```python
from build123d import *

# Parameters (mm, degrees)
SKETCH1_W             = 10
SKETCH1_H             = 15
BOSS_EXTRUDE1_DEPTH   = 15
M5X0_8_TAPPED_HOLE1_D = 4.2
M5X0_8_TAPPED_HOLE2_D = 4.2


with BuildPart() as part:
    # Sketch1 → Boss-Extrude1 (new body)
    with BuildSketch(Plane.XY):
        Rectangle(SKETCH1_W, SKETCH1_H)
    extrude(amount=BOSS_EXTRUDE1_DEPTH)

    # M5x0.8 Tapped Hole1 (through all)
    with Locations(Plane(origin=(0, 7.5, 0), x_dir=(1, 0, 0), z_dir=(0, 1, 0))):
        with Locations((0, -4)):
            Hole(M5X0_8_TAPPED_HOLE1_D / 2)

    # M5x0.8 Tapped Hole2 (through all)
    with Locations(Plane.ZY.offset(5)):
        with Locations((11, -2.5)):
            Hole(M5X0_8_TAPPED_HOLE2_D / 2)


solid = part.part
```
Here's how the part is built. I have some questions about the finished solid (model axes, mm). Give positions to 0.01 mm unless a question says otherwise; leave off trailing zeros. Order: outer loops, then holes, each group sorted by start corner. A loop starts at its lowest first (then second) coordinate and runs counter-clockwise, first axis right, second up. Notation, with made-up numbers: (31, -5.75) -> (90, -5.75) arc R14 ccw to (90, 16.25) -> close; hole circle Ø9 at (26, 8.5). An arc over 180 degrees is marked (long way). Use CSV: the item, a comma, the result in double quotes. Start each with the question number.
Item 1: Suppose I cut it at D-D (x = -2.5). List the corners of the cut face in (y, z) for me.
Item 2: Suppose I cut it at A-A (y = -2.5). List the corners of the cut face in (x, z) for me, and give its area (3 significant figures).
Item 3: If I drill on probe 1 along Y at (x, z) = (-0.5, 11); probe 2 along Z at (x, y) = (0, 0); probe 3 along Z at (x, y) = (0.5, -1), over which ranges is the centre line in solid material (lowest first)? Write a range as [from, to].
Item 4: Thinking about a two-plate mould opening in Z: for faces 1 (the flat face through (0, 0, 0)), 2 (the cylindrical face through (0.07, -2.41, 13.1)), 3 (the flat face through (0, 7.5, 7)), which applies, pulls with the +Z half, pulls with the -Z half, needs draft (parallel to the pull), parting line crosses it, or undercut?
Item 5: Suppose I cut it at B-B (z = 4). List the corners of the cut face in (x, y) for me, and give its area (3 significant figures).
Item 6: I'm going to push a flat-ended pin straight in: P1, Ø2, axis at x = -0.5, z = 4, coming from the +Y side. Where does the tip first touch, or does it pass through?
Item 7: Suppose I cut it at C-C (x = 0). List the corners of the cut face in (y, z) for me, and give its area (3 significant figures).
Answer block:
1,outline,"(-7.5, 0) -> (7.5, 0) -> (7.5, 15) -> (-7.5, 15) -> close; hole circle Ø4.2 at (-2.5, 11)"
2,outline,"(-5, 0) -> (5, 0) -> (5, 8.9) -> (-5, 8.9) -> close; (-5, 13.1) -> (5, 13.1) -> (5, 15) -> (-5, 15) -> close; hole circle Ø4.2 at (0, 4)"
2,area,"94.1 mm^2"
3,probe 1,"y = [-7.5, -4.6], [-0.4, 7.5]"
3,probe 2,"z = [0, 1.9], [6.1, 15]"
3,probe 3,"z = [0, 1.96], [6.04, 9.53], [12.47, 15]"
4,face 1,"pulls with the -Z half"
4,face 2,"undercut"
4,face 3,"needs draft"
5,outline,"(-5, -7.5) -> (-2.1, -7.5) -> (-2.1, 7.5) -> (-5, 7.5) -> close; (2.1, -7.5) -> (5, -7.5) -> (5, 7.5) -> (2.1, 7.5) -> close"
5,area,"87.0 mm^2"
6,P1,"passes through"
7,outline,"(-7.5, 0) -> (7.5, 0) -> (7.5, 1.9) -> (-7.5, 1.9) -> close; (-7.5, 6.1) -> (7.5, 6.1) -> (7.5, 15) -> (-7.5, 15) -> close; hole circle Ø4.2 at (-2.5, 11)"
7,area,"148 mm^2"
